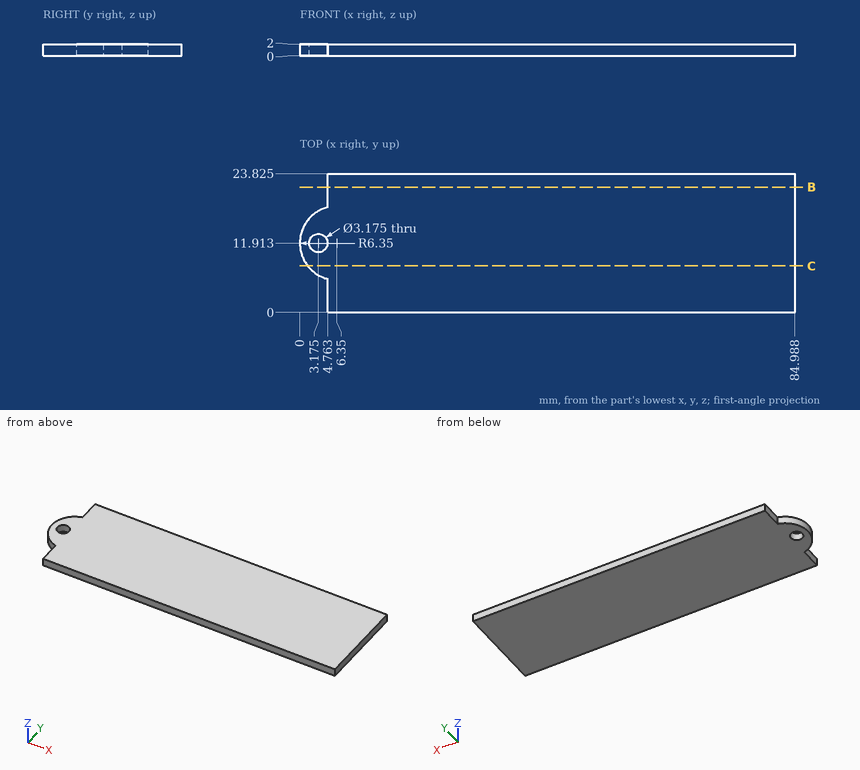
Verification items for this drawing (mm, ordinates from the low corner). Coordinates: 2 decimals unless noted, no trailing zeros. Order: outer loops, then holes, each group sorted by start corner. A loop starts at its lowest first (then second) coordinate and runs counter-clockwise, first axis right, second up.
Q1. Thickness scan on probe 1 along X at (y, z) = (5.75, 1.3) (1 decimal); probe 2 along Y at (x, z) = (4, 0.7) (1 decimal); probe 3 along X at (y, z) = (16, 1). Record the ranges inside material, lowest first.
Reply:
probe 1: x = 4.8 to 85
probe 2: y = 6 to 10.6, 13.3 to 17.8
probe 3: x = 1.49 to 84.99
Q2. Sectioned sample at B-B on y = 21.5. Record the cut outline in (x, z).
Reply:
outline: (4.76, 0) - (84.99, 0) - (84.99, 2) - (4.76, 2) - close
Q3. Sectioned sample at C-C on y = 8. Record the cut outline in (x, z).
Reply:
outline: (1.35, 0) - (84.99, 0) - (84.99, 2) - (1.35, 2) - close
